from build123d import *

# Parameters (mm, degrees)
SKETCH1_W           = 10.16
SKETCH1_H           = 10.5664
BOSS_EXTRUDE1_DEPTH = 1.27
SKETCH2_W           = 10.16
SKETCH2_H           = 8.89
BOSS_EXTRUDE2_DEPTH = 3.302
DRAFT1_ANGLE        = 5
EXTRUDE_THIN1_DEPTH = 0.4064
LPATTERN1_COUNT     = 5
LPATTERN1_PITCH     = 1.7018


with BuildPart() as part:
    # Sketch1 → Boss-Extrude1 (new body)
    with BuildSketch(Plane.XY):
        with Locations((5.08, 5.2832)):
            Rectangle(SKETCH1_W, SKETCH1_H)
    extrude(amount=BOSS_EXTRUDE1_DEPTH)

    # Sketch2 → Boss-Extrude2 (add)
    with BuildSketch(Plane.XY.offset(1.27)):
        with Locations((5.08, 4.445)):
            Rectangle(SKETCH2_W, SKETCH2_H)
    extrude(amount=BOSS_EXTRUDE2_DEPTH)

    # Draft1
    draft1_faces = [part.faces().sort_by_distance(p)[0] for p in [
        (5.08, 8.89, 2.921),
    ]]
    draft(draft1_faces, Plane.XY.offset(1.27), DRAFT1_ANGLE)

    # Sketch3 → Extrude-Thin1 (add, symmetric)
    with BuildSketch(Plane.ZY.offset(-1.6764)):
        with BuildLine():
            Line((2.286, 0), (2.286, -1.199738518))
            ThreePointArc((2.286, -1.199738518), (2.244995599, -1.338117976), (2.13522146, -1.431818957))
            Line((2.13522146, -1.431818957), (0.388422724, -2.208735427))
            ThreePointArc((0.388422724, -2.208735427), (0.081702678, -2.456965316), (-0.05973858, -2.825326055))
            Line((-0.05973858, -2.825326055), (-0.254, -4.6736))
            Line((-0.254, -4.6736), (0.251217123, -4.726700459))
            Line((0.251217123, -4.726700459), (0.445478542, -2.878426515))
            ThreePointArc((0.445478542, -2.878426515), (0.492625629, -2.755639602), (0.594865644, -2.672896305))
            Line((0.594865644, -2.672896305), (2.34166438, -1.895979835))
            ThreePointArc((2.34166438, -1.895979835), (2.670986798, -1.614876894), (2.794, -1.199738518))
            Line((2.794, -1.199738518), (2.794, 0))
            Line((2.794, 0), (2.286, 0))
        make_face()
    extrude_thin1 = extrude(amount=EXTRUDE_THIN1_DEPTH, both=True)

    # LPattern1: Extrude-Thin1 ×5
    with Locations(*[(i * LPATTERN1_PITCH, 0, 0) for i in range(1, LPATTERN1_COUNT)]):
        add(extrude_thin1)


solid = part.part
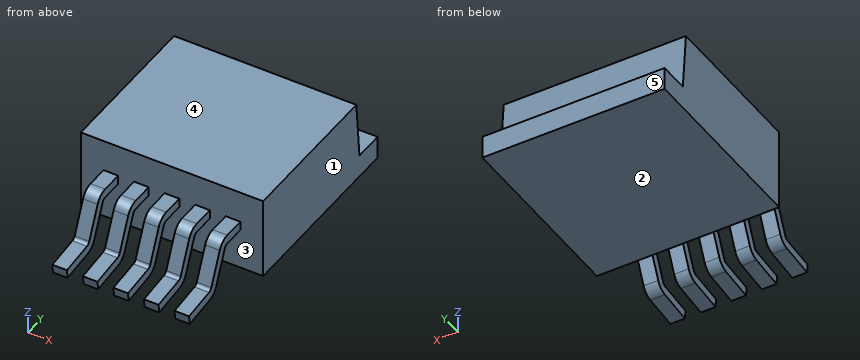
Here's how the part is built. I have some questions about the finished solid (model axes, mm). Face numbers are marked on the shaded views. A direction names the side the tool comes from. Round coordinates to 2 decimals unless told otherwise and drop trailing zeros. Loops run counter-clockwise (first coordinate to the right, second up) from the corner with the lowest first, then second, coordinate; pieces in that order, holes last.
1. If I drill on line 1 along Z through (x, y) = (3.75, 6); line 2 along Y through (x, z) = (6.5, 1.6); line 3 along Y through (x, z) = (4.5, 0.9), over which ranges is the centre line in solid material (lowest first)?
Answer list:
line 1: z = 0 to 4.57
line 2: y = -2.23 to -1.67, 0 to 8.86
line 3: y = 0 to 10.57
2. If we section it at A-A on x = 7.5: Write out the boundary of the cut face in (y, z), plus the area to 3 significant figures.
Answer list:
outline: (0, 0) - (10.57, 0) - (10.57, 1.27) - (8.89, 1.27) - (8.6, 4.57) - (0, 4.57) - close
area: 42.3 mm2
3. If we section it at D-D on y = 9.25: Write out the boundary of the cut face in (x, z).
Answer list:
outline: (0, 0) - (10.16, 0) - (10.16, 1.27) - (0, 1.27) - close
4. For P1, Ø1.5, axis at x = 6.5, z = 3, coming from the -Y side; P2, Ø2.5, axis at x = 4.5, z = 3, coming from the -Y side; P3, Ø1.5, axis at y = -1.5, z = 1, coming from the -X side, each with a flat end and sliding along its axis, tell me the tip position at first contact or that it passes through.
Answer list:
P1: stops at y = -1.94
P2: stops at y = -2.15
P3: stops at x = 1.27
5. We'd pull the mould along Y, two halves only. Please class the marked faces 3, 4 and 5: +Y half, -Y half, draft (parallel to the pull), parting line (faces both ways), or undercut.
Answer list:
face 3: undercut
face 4: draft
face 5: +Y half
6. If we section it at C-C on z = 1.05: Write out the boundary of the cut face in (x, y), plus the area to 3 significant figures.
Answer list:
outline: (0, 0) - (10.16, 0) - (10.16, 10.57) - (0, 10.57) - close; (1.27, -2.47) - (2.08, -2.47) - (2.08, -1.91) - (1.27, -1.91) - close; (2.97, -2.47) - (3.78, -2.47) - (3.78, -1.91) - (2.97, -1.91) - close; (4.67, -2.47) - (5.49, -2.47) - (5.49, -1.91) - (4.67, -1.91) - close; (6.38, -2.47) - (7.19, -2.47) - (7.19, -1.91) - (6.38, -1.91) - close; (8.08, -2.47) - (8.89, -2.47) - (8.89, -1.91) - (8.08, -1.91) - close
area: 110 mm2
7. Which directions (+Z, -Z, +X, -X, +Y, -Y) give clear straight access to the entire face, cutting with the end or side of a thin tool? Please do the marked faces 1 and 2.
Answer list:
face 1: +Z, -Z, +X, +Y, -Y
face 2: -Z, +X, -X, +Y
8. If we section it at B-B on y = -2.5: Write out the boundary of the cut face in (x, z), plus the area to 3 significant figures.
Answer list:
outline: (1.27, 0.05) - (2.08, 0.05) - (2.08, 0.98) - (1.27, 0.98) - close; (2.97, 0.05) - (3.78, 0.05) - (3.78, 0.98) - (2.97, 0.98) - close; (4.67, 0.05) - (5.49, 0.05) - (5.49, 0.98) - (4.67, 0.98) - close; (6.38, 0.05) - (7.19, 0.05) - (7.19, 0.98) - (6.38, 0.98) - close; (8.08, 0.05) - (8.89, 0.05) - (8.89, 0.98) - (8.08, 0.98) - close
area: 3.78 mm2
